Autodesk Inventor part; units mm, degrees
ref_plane "YZ Plane" through (0, 0, 0) normal (1, 0, 0) x (0, 1, 0)
ref_plane "XZ Plane" through (0, 0, 0) normal (0, 1, 0) x (-1, 0, 0)
ref_plane "XY Plane" through (0, 0, 0) normal (0, 0, 1) x (1, 0, 0)
sketch "Boceto1" plane through (0, 0, 0) normal (0, 1, 0) x (-1, 0, 0)
  line L0 (9.9, 20.3) -> (-9.9, 20.3)
  line L1 (-9.9, 20.3) -> (-9.9, -20.3)
  line L2 (-9.9, -20.3) -> (9.9, -20.3)
  line L3 (9.9, -20.3) -> (9.9, 20.3)
  line L4 (9.9, 20.3) -> (-9.9, -20.3) construction
  line L5 (-9.9, 20.3) -> (9.9, -20.3) construction
  point P0 (0, 0)
  dimension "d0" = 19.8
  dimension "d1" = 40.6
extrude "Extrusión1" add sketch "Boceto1" against normal blind 9
sketch "Boceto2" plane through (0, 0, 0) normal (0, 1, 0) x (1, 0, 0)
  circle A0 centre (0, 10.3) radius 3
  line L0 (9.9, 20.3) -> (-9.9, 20.3)
  point P0 (0, 0)
  dimension "d4" = 6
  dimension "d5" = 10
extrude "Extrusión2" cut sketch "Boceto2" against normal through all
sketch "Boceto5" plane through (0, -9, 0) normal (0, -1, 0) x (1, 0, 0)
  line L0 (-8.9, 20.3) -> (8.9, 20.3)
  line L1 (8.9, 20.3) -> (8.9, 27.3)
  line L2 (8.9, 27.3) -> (-8.9, 27.3)
  line L3 (-8.9, 27.3) -> (-8.9, 20.3)
  line L4 (-8.9, 20.3) -> (8.9, 27.3) construction
  line L5 (8.9, 20.3) -> (-8.9, 27.3) construction
  line L6 (-9.9, 27.3) -> (9.9, 27.3)
  line L7 (9.9, 20.3) -> (-9.9, 20.3)
  point P0 (0, 0)
  point P1 (0, 0)
  point P2 (0, 23.8)
  dimension "d23" = 17.8
  dimension "d24" = 7
extrude "Extrusión5" add sketch "Boceto5" against normal blind 2.8
sketch "Boceto6" plane through (0, -6.2, 0) normal (0, 1, 0) x (1, 0, 0)
  arc A0 (-3.75, -25.7967) -> (-6.25, -25.7967) centre (-5, -24.3) ccw
  line L0 (-8.9, -27.3) -> (8.9, -27.3)
  line L1 (-3.75, -27.3) -> (-6.25, -27.3)
  line L2 (-6.25, -27.3) -> (-6.25, -25.7967)
  line L3 (-3.75, -25.7967) -> (-3.75, -27.3)
  line L4 (0, -27.3) -> (0, -23.9124)
  line L5 (-8.9, -20.3) -> (-8.9, -27.3)
  line L6 (-8.9, -20.3) -> (8.9, -20.3)
  line L7 (-8.3229, -20.3) -> (8.9, -20.3)
  line L8 (8.9, -20.3) -> (8.9, -27.3)
  point P0 (0, 0)
  point P1 (0, 0)
  dimension "d27" = 3.9
  dimension "d28" = 3
  dimension "d29" = 5
  dimension "d75" = 1.25
  dimension "d76" = 1.25
extrude "Extrusión6" cut sketch "Boceto6" against normal through all contours L3 L0 L2 A0
sketch "Boceto8" plane through (0, 0, 0) normal (1, 0, 0) x (0, 1, 0)
  line L0 (-6.2, 27.3) -> (-5.4, 20.3)
  line L1 (-5.4, 20.3) -> (-6.2, 20.3)
  line L2 (-6.2, 20.3) -> (-6.2, 27.3)
  point P0 (0, 0)
  dimension "d34" = 0.8
extrude "Extrusión7" add sketch "Boceto8" along normal mid plane 1
mirror "Simetría3" about plane through (0, 0, 0) normal (1, 0, 0) of "Extrusión6"
mirror "Simetría4" about plane through (0, 0, 0) normal (0, 0, 1) of "Extrusión5", "Extrusión6", "Simetría3", "Extrusión7"
sketch "Boceto9" plane through (0, 0, 0) normal (0, 1, 0) x (1, 0, 0)
  circle A0 centre (0, 10.3) radius 3
  line L0 (-8.9, -13.5986) -> (8.9, -13.5986)
  line L1 (8.9, -13.5986) -> (8.9, 6.7014)
  line L2 (-8.9, 6.7014) -> (-8.9, -13.5986)
  line L3 (-8.9, -13.5986) -> (5.885, 8.9919) construction
  line L4 (8.9, -13.5986) -> (-5.885, 8.9919) construction
  arc A1 (8.9, 6.7014) -> (-8.9, 6.7014) centre (0, 10.3) ccw
  line L5 (9.9, 20.3) -> (-9.9, 20.3)
  point P0 (0, 0)
  dimension "d40" = 9.6
  dimension "d42" = 20.3
  dimension "d61" = 17.8
extrude "Extrusión8" add sketch "Boceto9" along normal blind 2
sketch "Boceto11" plane through (0, 2, 0) normal (0, 1, 0) x (1, 0, 0)
  line L0 (-8.9, -13.5986) -> (8.9, -13.5986)
  line L1 (5.2244, -15.7986) -> (5.2244, -13.5986)
  arc A0 (-4.1756, -13.5986) -> (5.2244, -13.5986) centre (0.5244, -9.6782) ccw
  line L2 (-4.1756, -13.5986) -> (5.2244, -13.5986)
  point P0 (0, 0)
  dimension "d50" = 2.2
  dimension "d51" = 9.4
extrude "Extrusión9" add sketch "Boceto11" against normal blind 2
sketch "Boceto12" plane through (0, 2, 0) normal (0, 1, 0) x (1, 0, 0)
  circle A0 centre (0, 10.3) radius 6.4
  circle A1 centre (0, 10.3) radius 3
  point P0 (0, 0)
  dimension "d54" = 12.8
extrude "Extrusión10" add sketch "Boceto12" along normal blind 1.3
sketch "Boceto13" plane through (0, 3.3, -10.3) normal (0, 1, 0) x (1, 0, 0)
  circle A0 centre (0, 0) radius 5.6
  circle A1 centre (0, 0) radius 3
  point P0 (0, -10.3)
  dimension "d57" = 11.2
extrude "Extrusión11" add sketch "Boceto13" along normal blind 0.9
sketch "Boceto15" plane through (0, 2, 0) normal (0, 1, 0) x (1, 0, 0)
  line L0 (8.9, 6.7014) -> (8.9, -13.5986)
  line L1 (-8.9, -13.5986) -> (8.9, -13.5986)
  line L2 (8.9, -13.5986) -> (8.9, -1.0986)
  line L3 (8.9, -1.0986) -> (-8.9, -1.0986)
  line L4 (-8.9, -1.0986) -> (-8.9, -13.5986)
  line L5 (-8.9, -13.5986) -> (8.9, -1.0986) construction
  line L6 (8.9, -13.5986) -> (-8.9, -1.0986) construction
  line L7 (-8.9, -13.5986) -> (-4.1756, -13.5986)
  line L8 (-7.8, -12.4986) -> (7.8, -12.4986)
  line L9 (7.8, -12.4986) -> (7.8, -2.1986)
  line L10 (7.8, -2.1986) -> (-7.8, -2.1986)
  line L11 (-7.8, -2.1986) -> (-7.8, -12.4986)
  point P0 (0, 0)
  point P1 (0, -7.3486)
  dimension "d62" = 12.5
  dimension "d63" = 1.1
extrude "Extrusión12" add sketch "Boceto15" along normal blind 0.3
sketch "Boceto16" plane through (0, 2.3, 0) normal (0, 1, 0) x (1, 0, 0)
  arc A0 (1.91, -1.0986) -> (-1.91, -1.0986) centre (0, -0.7586) ccw
  line L0 (-7.8, -2.1986) -> (7.8, -2.1986)
  line L1 (8.9, -1.0986) -> (-8.9, -1.0986)
  point P0 (0, 0)
  dimension "d66" = 3.88
  dimension "d67" = 1.44
extrude "Extrusión13" add sketch "Boceto16" against normal blind 0.3
sketch "Boceto17" plane through (0, 0, 0) normal (0, 1, 0) x (1, 0, 0)
  line L0 (-9.9, 20.3) -> (-9.9, -20.3)
  line L1 (9.9, -20.3) -> (9.9, 20.3)
  line L2 (-9.9, -20.3) -> (9.9, -20.3)
  line L3 (9.9, 20.3) -> (-9.9, 20.3)
  line L4 (-9.6, -20) -> (-9.6, 20)
  line L5 (-9.6, 20) -> (9.6, 20)
  line L6 (9.6, 20) -> (9.6, -20)
  line L7 (9.6, -20) -> (-9.6, -20)
  point P0 (0, 0)
  dimension "d70" = 0.3
extrude "Extrusión14" cut sketch "Boceto17" against normal blind 0.5
fillet "Empalme1" radius 1 10 edges at (9.9, -4.75, 20.3) (8.9, -7.6, 27.3) (-8.9, -7.6, 27.3) (-9.9, -4.75, 20.3) (8.9, 1.15, 13.5986) (-8.9, 1.15, 13.5986) (9.9, -4.75, -20.3) (-9.9, -4.75, -20.3) (-8.9, -7.6, -27.3) (8.9, -7.6, -27.3)
fillet "Empalme2" radius 0.7 4 edges at (9.6, -0.25, 20) (-9.6, -0.25, 20) (9.6, -0.25, -20) (-9.6, -0.25, -20)
sketch "Boceto18" plane through (0, 2, 0) normal (0, 1, 0) x (1, 0, 0)
  point P0 (0, 0)
equation "\"d76\" = d75"
properties part number "Top" material "Plástico ABS"
Verification items for the finished model (mm, model axes). A direction names the side the tool comes from. Coordinates: 2 decimals unless noted, no trailing zeros. Order: outer loops, then holes, each group sorted by start corner. A loop starts at its lowest first (then second) coordinate and runs counter-clockwise, first axis right, second up. Notation, with made-up numbers: (69.25, 75) -> (73.25, 75) arc R22 ccw to (73.25, 101) -> close; hole circle Ø1 at (65.5, 43.25). An arc over 180 degrees is marked (long way). Answer as CSV lines item,"result". Start each with the question number.
1) Cross-section at A-A, the plane y = -4.5. Record the boundary of the cut face in (x, z), then the cut area to 3 significant figures.
2) Gauge pin test, flat ends, axial feed: pin 1 Ø1.8 at (y, z) = (1, 4.5) entering from -X; pin 2 Ø0.5 at (y, z) = (-8, -26.5) entering from +X; pin 3 Ø0.6 at (y, z) = (-5.5, -22) entering from -X. Record the tip position at first contact, or that the pin passes through.
3) Set-up check for faces 1 (the face through (-7, -8, 27.3)), 2 (the face through (2.9, 0, -19.8)), 3 (the face through (0, -9, 0)), 4 (the face through (5, -6.2, 22)), 5 (the face through (-0.263, 0.986, -19.896)): record each of +Z, -Z, +X, -X, +Y, -Y from which the full face is reachable in a straight line by a thin tool's end or side.
4) Cross-section at C-C, the plane z = 0. Record the boundary of the cut face in (x, y), then the cut area to 3 significant figures.
5) Release check for a two-part mould opening along X. For faces 6 (the face through (-9.9, -5, 0)), 7 (the face through (8.599, -7.58, 27.015)), 8 (the face through (-3.75, -8, -27)), 9 (the face through (3.75, -8, -27)) record: released by +X, released by -X, zero draft, split by the parting line, or undercut.
6) Cross-section at B-B, the plane z = 24.3. Record the boundary of the cut face in (x, y), then the cut area to 3 significant figures.
7) Material ranges on L1, parallel to X at y = -7.3, z = -24.3; L2, parallel to X at y = -4, z = -10.3; L3, parallel to Y at x = 2.75, z = 19, recorded low to high. Write a range as [from, to].
Conclusion:
1,outline,"(-9.9, -19.3) arc R1 ccw to (-8.9, -20.3) -> (8.9, -20.3) arc R1 ccw to (9.9, -19.3) -> (9.9, 19.3) arc R1 ccw to (8.9, 20.3) -> (-8.9, 20.3) arc R1 ccw to (-9.9, 19.3) -> close; hole circle Ø6 at (0, -10.3)"
1,area,"775 mm²"
2,pin 1,"stops at x = -8.9"
2,pin 2,"stops at x = 8.9"
2,pin 3,"stops at x = -0.5"
3,face 1,"+Z, +X, -X, +Y, -Y"
3,face 2,"-Z, +Y"
3,face 3,"+Z, -Z, +X, -X, -Y"
3,face 4,"+Z, +X, +Y"
3,face 5,"+Y"
4,outline,"(-9.9, -9) -> (9.9, -9) -> (9.9, -0.5) -> (9.6, -0.5) -> (9.6, 0) -> (8.9, 0) -> (8.9, 2) -> (1.79, 2) -> (1.79, 2.3) -> (-1.79, 2.3) -> (-1.79, 2) -> (-8.9, 2) -> (-8.9, 0) -> (-9.6, 0) -> (-9.6, -0.5) -> (-9.9, -0.5) -> close"
4,area,"215 mm²"
5,face 6,"released by -X"
5,face 7,"released by +X"
5,face 8,"undercut"
5,face 9,"undercut"
6,outline,"(-8.9, -9) -> (-6.95, -9) -> (-6.95, -6.2) -> (-8.9, -6.2) -> close; (-3.05, -9) -> (3.05, -9) -> (3.05, -6.2) -> (0.5, -6.2) -> (0.5, -5.86) -> (-0.5, -5.86) -> (-0.5, -6.2) -> (-3.05, -6.2) -> close; (6.95, -9) -> (8.9, -9) -> (8.9, -6.2) -> (6.95, -6.2) -> close"
6,area,"28.3 mm²"
7,L1,"x = [-8.9, -6.95], [-3.05, 3.05], [6.95, 8.9]"
7,L2,"x = [-9.9, -3], [3, 9.9]"
7,L3,"y = [-9, 0]"
